```python
from build123d import *

# Parameters (mm, degrees)
SKETCH1_R               = 6
BOSS_EXTRUDE1_DEPTH     = 30
SKETCH2_R               = 3.175
CUT_EXTRUDE1_DEPTH      = 1
CUT_EXTRUDE1_DEPTH_BACK = 31
SKETCH4_R               = 1.5
CUT_EXTRUDE4_DEPTH      = 7
CUT_EXTRUDE4_DEPTH_BACK = 7


with BuildPart() as part:
    # Sketch1 → Boss-Extrude1 (new body)
    with BuildSketch(Plane(origin=(0, 0, 0), x_dir=(1, 0, 0), z_dir=(0, 1, 0))):
        Circle(SKETCH1_R)
    extrude(amount=BOSS_EXTRUDE1_DEPTH)

    # Sketch2 → Cut-Extrude1 (cut, two sides)
    with BuildSketch(Plane(origin=(0, 30, 0), x_dir=(1, 0, 0), z_dir=(0, 1, 0))) as cut_extrude1_sk:
        Circle(SKETCH2_R)
    extrude(amount=CUT_EXTRUDE1_DEPTH, mode=Mode.SUBTRACT)
    extrude(cut_extrude1_sk.sketch, amount=-CUT_EXTRUDE1_DEPTH_BACK, mode=Mode.SUBTRACT)

    # Sketch4 → Cut-Extrude4 (cut, two sides)
    with BuildSketch(Plane.XY) as cut_extrude4_sk:
        with Locations((0, 25)):
            Circle(SKETCH4_R)
        with Locations((0, 5)):
            Circle(SKETCH4_R)
    extrude(amount=CUT_EXTRUDE4_DEPTH, mode=Mode.SUBTRACT)
    extrude(cut_extrude4_sk.sketch, amount=-CUT_EXTRUDE4_DEPTH_BACK, mode=Mode.SUBTRACT)


solid = part.part
```
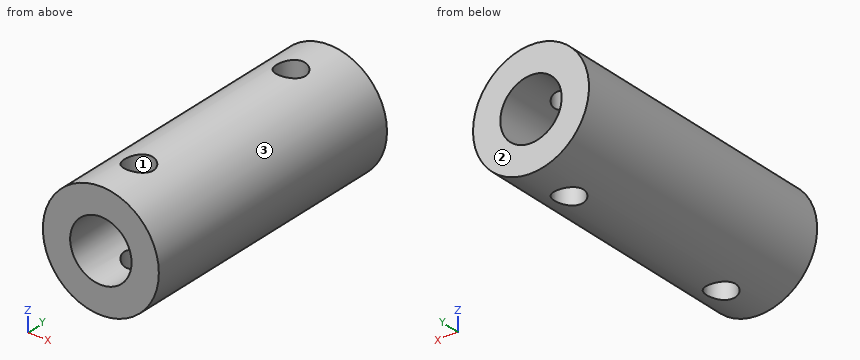
Check sheet for the modelled part. Datum: model origin and axes. Units: mm. Face numbers are marked on the shaded views. Round coordinates to 2 decimals unless told otherwise and drop trailing zeros. Loops run counter-clockwise (first coordinate to the right, second up) from the corner with the lowest first, then second, coordinate; pieces in that order, holes last. Notation, with made-up numbers: (-37, 50) - (22, 50) arc R33 ccw to (22, 84) - close; hole circle Ø9 at (-3, -11). An arc over 180 degrees is marked (long way). Answer as a JSON object with one key per item and string values. Group by question number.
Q1. Sectioned sample at D-D, the plane z = 4.75. Enter the section's corners in (x, y), plus the area to 3 significant figures.
Q2. Gauge pin test, flat ends, axial feed: P1, Ø1.8, axis at x = 0, y = 25, coming from the +Z side; P2, Ø5, axis at x = 3.5, y = 26, coming from the +Z side. Record the tip position at first contact, or that the pin passes through.
Q3. Sectioned sample at C-C, the plane y = 5. Enter the section's corners in (x, z) (3 decimals).
Q4. Mould release check, pull along X, two halves, no side actions. Record for the marked faces 1, 2 and 3: released by +X, released by -X, zero draft, split by the parting line, or undercut.
Q5. Scan lines: line 1 along Y through (x, z) = (0, 4.5); line 2 along X through (y, z) = (9, 0) (3 decimals). Record each from-to range of solid material in increasing order. Write a range as [from, to].
Q6. Sectioned sample at A-A, the plane x = 0. Enter the section's corners in (y, z) (3 decimals).
Q7. Sectioned sample at B-B, the plane z = 0. Enter the section's corners in (x, y) (3 decimals).
Solution:
{
 "1": {"outline": "(-3.67, 0) - (3.67, 0) - (3.67, 30) - (-3.67, 30) - close; hole circle Ø3 at (0, 5); hole circle Ø3 at (0, 25)", "area": "206 mm²"},
 "2": {"P1": "passes through", "P2": "stops at z = 5.92"},
 "3": {"outline": "(-1.5, -5.809) - (-1.5, -2.798) arc R3.175 cw to (-1.5, 2.798) - (-1.5, 5.809) arc R6 ccw to start; (1.5, -5.809) arc R6 ccw to (1.5, 5.809) - (1.5, 2.798) arc R3.175 cw to (1.5, -2.798) - close"},
 "4": {"face 1": "undercut", "face 2": "zero draft", "face 3": "split by the parting line"},
 "5": {"line 1": "y = [0, 3.5], [6.5, 23.5], [26.5, 30]", "line 2": "x = [-6, -3.175], [3.175, 6]"},
 "6": {"outline": "(0, -6) - (3.5, -6) - (3.5, -3.175) - (0, -3.175) - close; (0, 3.175) - (3.5, 3.175) - (3.5, 6) - (0, 6) - close; (6.5, -6) - (23.5, -6) - (23.5, -3.175) - (6.5, -3.175) - close; (6.5, 3.175) - (23.5, 3.175) - (23.5, 6) - (6.5, 6) - close; (26.5, -6) - (30, -6) - (30, -3.175) - (26.5, -3.175) - close; (26.5, 3.175) - (30, 3.175) - (30, 6) - (26.5, 6) - close"},
 "7": {"outline": "(-6, 0) - (-3.175, 0) - (-3.175, 30) - (-6, 30) - close; (3.175, 0) - (6, 0) - (6, 30) - (3.175, 30) - close"}
}
